CAD build for the part. Positions are in the model's coordinates, mm. A direction names the side the tool comes from. Round coordinates to 2 decimals unless told otherwise and drop trailing zeros. Write each loop counter-clockwise with the first axis right and the second up, starting at its lowest first coordinate (ties: lowest second). Pieces come first, ordered by that corner, then holes. Notation, with made-up numbers: (-11.75, 62) - (35.25, 62) arc R21 cw to (35.25, 67) - close; hole circle Ø7 at (3.25, -40). An arc over 180 degrees is marked (long way). Use one line per item in the form item = value. Start each with the question number.
Item 1: Band-saw the part on A-A, the plane x = 20.5. List the corners of the cut face in (y, z), and give its area (3 significant figures).
Item 2: Drill centre lines: L1, parallel to Y at x = 15, z = -295; L2, parallel to X at y = -181, z = -68.5; L3, parallel to Z at x = 17.5, y = -213. Where is each one in solid material? Low to high.
Item 3: Pin check, flat tips, straight feed: pin 1 (1.1 mm diameter, centred on x = 12, y = -0.5, fed in from +Z); pin 2 (6 mm diameter, centred on x = 22, y = -123, fed in from +Z); pin 3 (1.1 mm diameter, centred on y = -246.5, z = -134.5, fed in from +X). Stop position of each tip, or through.
Item 4: Band-saw the part on C-C, the plane z = -192. List the corners of the cut face in (x, y).
Item 5: Tool access for faces 4 (the flat face through (-1.122, -122, -112)), 5 (the flat face through (12, -246, -113)): list every direction of +Z, -Z, +X, -X, +Y, -Y with a clear straight run to the whole face (end or side of a thin tool).
Item 6: Pull direction Y, two halves, no side cores. Call faces 1 (the flat face through (14, 0, -113)), 2 (the flat face through (13.79, -121.77, -307.73)), 3 (the flat face through (12, -1, -113)): +Y half, -Y half, draft (parallel to the pull), parting line (faces both ways), or undercut.
Item 7: Band-saw the part on B-B, the plane y = -71. List the corners of the cut face in (x, z).
from build123d import *

# Parameters (mm, degrees)
F1_DEPTH = 247
F2_W     = 25
F2_H     = 1
F3_DEPTH = 1
F2_H_2   = 374
F4_DEPTH = 1
F6_DEPTH = 1


# Not quite as in the source:
# - a feature names something its author has since deleted; it is built from what else it names


with BuildPart() as f1:
    # F0 (on Front) → F1 (new body)
    with BuildSketch(Plane.XZ):
        Polygon((-1.1216281516, 73.3666580543), (-1.1216281516, 72.3666580543), (-1.1216281516, -302.6333419457), (-1.1216281516, -303.6333419457), (29.1284304133, -311.9432493216), (29.1284304133, -310.9432493216), (0, -303.1383099156), (0, 71.8616900844), (27.561313438, 79.2467217624), (27.3271471585, 80.2189183236), align=None)
    extrude(amount=F1_DEPTH)

    # F2 (on Front) → F3 (join)
    with BuildSketch(Plane.XZ):
        with Locations((12.390091487, 71.8666580543)):
            Rectangle(F2_W, F2_H)
    extrude(amount=F3_DEPTH)

    # F2 (on Front) → F4 (join)
    with BuildSketch(Plane.XZ):
        with Locations((12.390091487, -115.6333419457)):
            Rectangle(F2_W, F2_H_2)
    extrude(amount=F4_DEPTH)

    # F5 (on face) → F6 (join)
    with BuildSketch(Plane.XZ.offset(247)):
        Polygon((24.5685894042, 71.8616900844), (0, 71.8616900844), (0, -303.1383099156), (24.5685894042, -302.4606704712), align=None)
    extrude(amount=-F6_DEPTH)


solid = f1.part
Determined:
q1.outline = (-247, -309.57) - (0, -309.57) - (0, -308.63) - (-247, -308.63) - close; (-247, -302.57) - (-246, -302.57) - (-246, 71.86) - (-247, 71.86) - close; (-247, 77.35) - (0, 77.35) - (0, 78.57) - (-247, 78.57) - close; (-1, -302.63) - (0, -302.63) - (0, 72.37) - (-1, 72.37) - close
q1.area = 1,280 mm²
q2.L1 = -247 to -246, -1 to 0
q2.L2 = -1.12 to 0
q2.L3 = -308.75 to -307.83, 76.55 to 77.85
q3.pin_1 = 76.66
q3.pin_2 = 79.66
q3.pin_3 = 24.57
q4.outline = (-1.12, -247) - (24.57, -247) - (24.57, -246) - (0, -246) - (0, -1) - (24.89, -1) - (24.89, 0) - (-1.12, 0) - close
q5.face_4 = +Z, -Z, -X, +Y, -Y
q5.face_5 = +X
q6.face_1 = +Y half
q6.face_2 = draft
q6.face_3 = undercut
q7.outline = (-1.12, -303.63) - (29.13, -311.94) - (29.13, -310.94) - (0, -303.14) - (0, 71.86) - (27.56, 79.25) - (27.33, 80.22) - (-1.12, 73.37) - close
